Here's how the part is built. I have some questions about the finished solid (model axes, mm). Face numbers are marked on the shaded views. Give positions to 0.01 mm unless a question says otherwise; leave off trailing zeros. Order: outer loops, then holes, each group sorted by start corner. A loop starts at its lowest first (then second) coordinate and runs counter-clockwise, first axis right, second up. Notation, with made-up numbers: (56, 53) -> (71, 53) arc R35 cw to (71, 87) -> close; hole circle Ø3 at (15.5, -16). An arc over 180 degrees is marked (long way). Write each question's results on one line, items separated by ' | '. Start each with the question number.
Q1. I need wall thicknesses on line 1 along Y through (x, z) = (0, 8); line 2 along Y through (x, z) = (29, 3.25); line 3 along X through (y, z) = (3, 3.25). Which ranges of each line are inside material? Lowest first, please. Write a range as [from, to].
Q2. Imagine slicing it at C-C, the plane z = 2.75. Please give me the cut outline in (x, y), then the cut area to 3 significant figures.
Q3. Imagine slicing it at B-B, the plane x = 25. Please give me the cut outline in (y, z), then the cut area to 3 significant figures.
Q4. I'm going to push flat-ended pins straight in: pin 1 (6 mm diameter, centred on x = 10, y = -7.5, fed in from -Z); pin 2 (6 mm diameter, centred on y = 2, z = 3, fed in from +X); pin 3 (2 mm diameter, centred on x = -3, z = 6.5, fed in from +Y); pin 4 (18 mm diameter, centred on x = 25, y = 0, fed in from +Z). Where does each tip first touch, or does it pass through?
Q5. Imagine slicing it at A-A, the plane y = 0. Please give me the cut outline in (x, z), then the cut area to 3 significant figures.
Q6. Thinking about a two-plate mould opening in X: for the marked faces 1, 2 and 3, which applies, pulls with the +X half, pulls with the -X half, needs draft (parallel to the pull), parting line crosses it, or undercut?
Q7. Imagine slicing it at D-D, the plane y = 12.5. Please give me the cut outline in (x, z), then the cut area to 3 significant figures.
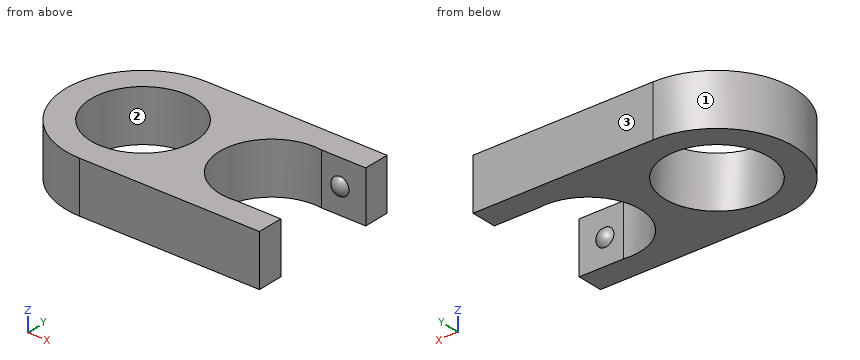
```python
from build123d import *

# Parameters (mm, degrees)
CYLINDER002_R     = 10.1
CYLINDER002_DEPTH = 10
BOX001_W          = 10
BOX001_H          = 20
BOX001_DEPTH      = 10
CYLINDER001_R     = 10.1
CYLINDER001_DEPTH = 10
BOX_W             = 35
BOX_H             = 30
BOX_DEPTH         = 10
CYLINDER_R        = 15
CYLINDER_DEPTH    = 10


with BuildPart() as sphere:
    # Sphere → Sphere (revolve)
    with BuildSketch(Plane(origin=(30, 11, 5), x_dir=(1, 0, 0), z_dir=(0, -1, 0))):
        with BuildLine():
            ThreePointArc((0, -2), (2, 0), (0, 2))
            Line((0, 2), (0, -2))
        make_face()
    revolve(axis=Axis((30, 11, 5), (0, 0, 1)))


with BuildPart() as cylinder002:
    # Cylinder002 → Cylinder002 (new body)
    with BuildSketch(Plane(origin=(25, 0, 0), x_dir=(1, 0, 0), z_dir=(0, 0, 1))):
        Circle(CYLINDER002_R)
    extrude(amount=CYLINDER002_DEPTH)


with BuildPart() as cube001:
    # Box001 → Box001 (new body)
    with BuildSketch(Plane(origin=(25, -10, 0), x_dir=(1, 0, 0), z_dir=(0, 0, 1))):
        with Locations((5, 10)):
            Rectangle(BOX001_W, BOX001_H)
    extrude(amount=BOX001_DEPTH)


with BuildPart() as negative_fusion:
    # Cylinder001 → Cylinder001 (new body)
    with BuildSketch(Plane.XY):
        Circle(CYLINDER001_R)
    extrude(amount=CYLINDER001_DEPTH)

    # Fusion001: union Cylinder002, Cube001
    add(cylinder002.part)
    add(cube001.part)


with BuildPart() as cube:
    # Box → Box (new body)
    with BuildSketch(Plane(origin=(0, -15, 0), x_dir=(1, 0, 0), z_dir=(0, 0, 1))):
        with Locations((17.5, 15)):
            Rectangle(BOX_W, BOX_H)
    extrude(amount=BOX_DEPTH)


with BuildPart() as cut:
    # Cylinder → Cylinder (new body)
    with BuildSketch(Plane.XY):
        Circle(CYLINDER_R)
    extrude(amount=CYLINDER_DEPTH)

    # Fusion: union Cube
    add(cube.part)

    # Cut: cut Negative Fusion
    add(negative_fusion.part, mode=Mode.SUBTRACT)


with BuildPart() as fusion002:
    # Sphere001 → Sphere001 (revolve)
    with BuildSketch(Plane(origin=(30, -11, 5), x_dir=(1, 0, 0), z_dir=(0, -1, 0))):
        with BuildLine():
            ThreePointArc((0, -2), (2, 0), (0, 2))
            Line((0, 2), (0, -2))
        make_face()
    revolve(axis=Axis((30, -11, 5), (0, 0, 1)))

    # Fusion002: union Sphere, Cut
    add(sphere.part)
    add(cut.part)


solid = fusion002.part
```
Geometry check:
1) line 1: [-15, -10.1], [10.1, 15] | line 2: [-15, -10], [10, 15] | line 3: [-14.7, -9.64], [9.64, 15.36]
2) outline: (0, -15) -> (35, -15) -> (35, -10) -> (26.42, -10) arc R10.1 cw (long way) to (26.42, 10) -> (35, 10) -> (35, 15) -> (0, 15) arc R15 ccw to start; hole circle Ø20.2 at (0, 0) | area: 723 mm²
3) outline: (-15, 0) -> (-10.1, 0) -> (-10.1, 10) -> (-15, 10) -> close; (10.1, 0) -> (15, 0) -> (15, 10) -> (10.1, 10) -> close | area: 98.0 mm²
4) pin 1: z = 0 | pin 2: x = 16.22 | pin 3: y = 14.87 | pin 4: through
5) outline: (-15, 0) -> (-10.1, 0) -> (-10.1, 10) -> (-15, 10) -> close; (10.1, 0) -> (14.9, 0) -> (14.9, 10) -> (10.1, 10) -> close | area: 97.0 mm²
6) face 1: pulls with the -X half | face 2: undercut | face 3: needs draft
7) outline: (-8.29, 0) -> (35, 0) -> (35, 10) -> (-8.29, 10) -> close | area: 433 mm²
